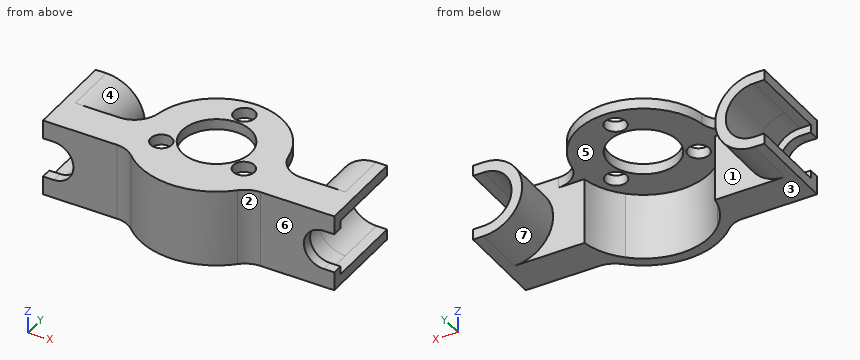
from build123d import *

# Parameters (mm, degrees)
BOSS_EXTRU_1_DEPTH      = 7
BOSS_EXTRU_3_DEPTH      = 2
ESQUISSE2_RX            = 12.5
ESQUISSE2_RY            = 12.5
ENL_V_MAT_EXTRU_1_DEPTH = 40.69604363
ESQUISSE3_R             = 12.5
ESQUISSE3_R_2           = 6.5
ESQUISSE3_R_3           = 2
BOSS_EXTRU_2_DEPTH      = 2
BOSS_EXTRU_4_DEPTH      = 14.56
CONG_2_R                = 5
BOSS_EXTRU_5_DEPTH      = 10


with BuildPart() as part:
    # Esquisse1 → Boss.-Extru.1 (new body)
    with BuildSketch(Plane(origin=(0, 0, 0), x_dir=(1, 0, 0), z_dir=(0, 1, 0))):
        with BuildLine():
            Line((36.259926639, -6.254535912), (36.259926639, -8.254535912))
            Line((36.259926639, -8.254535912), (28.259926639, -8.254535912))
            Line((28.259926639, -8.254535912), (26.259926639, -8.254535912))
            Line((26.259926639, -8.254535912), (-8.740073361, -8.254535912))
            Line((-8.740073361, -8.254535912), (-10.740073361, -8.254535912))
            Line((-10.740073361, -8.254535912), (-18.740073361, -8.254535912))
            Line((-18.740073361, -8.254535912), (-18.740073361, -6.254535912))
            Line((-18.740073361, -6.254535912), (-16.740073361, -6.254535912))
            ThreePointArc((-16.740073361, -6.254535912), (-13.378645093, -5.04629229), (-11.555635108, -1.974535912))
            ThreePointArc((-11.555635108, -1.974535912), (-11.460073361, -0.974535912), (-11.555635108, 0.025464088))
            ThreePointArc((-11.555635108, 0.025464088), (-13.378645093, 3.097220466), (-16.740073361, 4.305464088))
            Line((-16.740073361, 4.305464088), (-18.740073361, 4.305464088))
            Line((-18.740073361, 4.305464088), (-18.740073361, 6.305464088))
            Line((-18.740073361, 6.305464088), (-10.740073361, 6.305464088))
            Line((-10.740073361, 6.305464088), (-8.740073361, 6.305464088))
            Line((-8.740073361, 6.305464088), (26.259926639, 6.305464088))
            Line((26.259926639, 6.305464088), (28.259926639, 6.305464088))
            Line((28.259926639, 6.305464088), (36.259926639, 6.305464088))
            Line((36.259926639, 6.305464088), (36.259926639, 4.305464088))
            Line((36.259926639, 4.305464088), (34.259926639, 4.305464088))
            ThreePointArc((34.259926639, 4.305464088), (30.898498371, 3.097220466), (29.075488386, 0.025464088))
            ThreePointArc((29.075488386, 0.025464088), (28.979926639, -0.974535912), (29.075488386, -1.974535912))
            ThreePointArc((29.075488386, -1.974535912), (30.898498371, -5.04629229), (34.259926639, -6.254535912))
            Line((34.259926639, -6.254535912), (36.259926639, -6.254535912))
        make_face()
    extrude(amount=BOSS_EXTRU_1_DEPTH)

    # Esquisse4 → Boss.-Extru.3 (add)
    with BuildSketch(Plane.XZ):
        with BuildLine():
            Line((34.259926639, 4.724535912), (36.259926639, 4.724535912))
            Line((36.259926639, 4.724535912), (36.259926639, 6.254535912))
            Line((36.259926639, 6.254535912), (34.259926639, 6.254535912))
            ThreePointArc((34.259926639, 6.254535912), (28.979926639, 0.974535912), (34.259926639, -4.305464088))
            Line((34.259926639, -4.305464088), (36.259926639, -4.305464088))
            Line((36.259926639, -4.305464088), (36.259926639, -2.775464088))
            Line((36.259926639, -2.775464088), (34.259926639, -2.775464088))
            ThreePointArc((34.259926639, -2.775464088), (30.509926639, 0.974535912), (34.259926639, 4.724535912))
        make_face()
        with BuildLine():
            Line((-18.740073361, -2.775464088), (-18.740073361, -4.305464088))
            Line((-18.740073361, -4.305464088), (-16.740073361, -4.305464088))
            ThreePointArc((-16.740073361, -4.305464088), (-11.460073361, 0.974535912), (-16.740073361, 6.254535912))
            Line((-16.740073361, 6.254535912), (-18.740073361, 6.254535912))
            Line((-18.740073361, 6.254535912), (-18.740073361, 4.724535912))
            Line((-18.740073361, 4.724535912), (-16.740073361, 4.724535912))
            ThreePointArc((-16.740073361, 4.724535912), (-12.990073361, 0.974535912), (-16.740073361, -2.775464088))
            Line((-16.740073361, -2.775464088), (-18.740073361, -2.775464088))
        make_face()
    extrude(amount=-BOSS_EXTRU_3_DEPTH)

    # Esquisse2 → Enl_v. mat.-Extru.1 (cut, through all)
    with BuildSketch(Plane.XY.offset(8.254535912)):
        with Locations(Location((8.759926639, 9), (0, 0, 180))):
            Ellipse(ESQUISSE2_RX, ESQUISSE2_RY)
    extrude(amount=-ENL_V_MAT_EXTRU_1_DEPTH, mode=Mode.SUBTRACT)


with BuildPart() as enl_v_mat_extru_1_piece_1:
    # of the separate pieces the step leaves, piece 1, a body of its own (enl_v_mat_extru_1_pieces)
    add(part.part.solids().sort_by_distance((-18.740073361, 7, -6.305464088))[0])

    # Esquisse3 → Boss.-Extru.2 (add)
    with BuildSketch(Plane.XY.offset(8.254535912)):
        with Locations((8.759926639, 9)):
            Circle(ESQUISSE3_R)
        with Locations((8.759926639, 9)):
            Circle(ESQUISSE3_R_2, mode=Mode.SUBTRACT)
        with Locations((8.759926639, 18)):
            Circle(ESQUISSE3_R_3, mode=Mode.SUBTRACT)
        with Locations((16.554155273, 4.5)):
            Circle(ESQUISSE3_R_3, mode=Mode.SUBTRACT)
        with Locations((0.965698005, 4.5)):
            Circle(ESQUISSE3_R_3, mode=Mode.SUBTRACT)
    extrude(amount=-BOSS_EXTRU_2_DEPTH)



with BuildPart() as enl_v_mat_extru_1_piece_2:
    # of the separate pieces the step leaves, piece 2, a body of its own (enl_v_mat_extru_1_pieces)
    add(part.part.solids().sort_by_distance((34.259926639, 2, 6.254535912))[0])


with BuildPart() as enl_v_mat_extru_1_piece_1_1:
    add(enl_v_mat_extru_1_piece_1.part)

    add(enl_v_mat_extru_1_piece_2.part)  # Boss.-Extru.4 merges Enl_v. mat.-Extru.1 piece 2
    # Esquisse6 → Boss.-Extru.4 (add)
    with BuildSketch(Plane.XY.offset(8.254535912)):
        with BuildLine():
            Line((0.085250852, 0), (-2.608890362, 0))
            ThreePointArc((-2.608890362, 0), (8.759926639, -5.5), (20.12874364, 0))
            Line((20.12874364, 0), (17.434602425, 0))
            ThreePointArc((17.434602425, 0), (8.759926639, -3.5), (0.085250852, 0))
        make_face()
    extrude(amount=-BOSS_EXTRU_4_DEPTH)

    # Cong_2
    # the kernel refuses this fillet: 5 mm, written as the material it adds along each edge
    with BuildSketch(Plane(origin=(20.12874364, 0, 8.254535912), x_dir=(1, 0, 0), z_dir=(0, 0, -1))) as cong_2_piece_1:
        with BuildLine():
            CenterArc((2.20505496, 5), CONG_2_R, 225.885381452, 44.114618548)
            ThreePointArc((-1.27542503, 1.41025641), (-0.614570897, 0.726057307), (0, 0))
            Line((0, 0), (2.20505496, 0))
        make_face()
    extrude(amount=14.56)
    with BuildSketch(Plane(origin=(-2.608890362, 0, 8.254535912), x_dir=(0.6707625728642448, -0.7416721451184065, 0), z_dir=(0, 0, -1))) as cong_2_piece_2:
        with BuildLine():
            CenterArc((2.229292388, 4.989240706), CONG_2_R, 222.125947854, 44.114618548)
            Line((-1.479068338, 1.635427842), (0, 0))
            ThreePointArc((0, 0), (0.950727636, 0.031201952), (1.901455272, 0))
        make_face()
    extrude(amount=14.56)
    with BuildSketch(Plane(origin=(21.098889318, 7, 6.254535912), x_dir=(1, 0, 0), z_dir=(0, 0, 1))) as cong_2_piece_3:
        with BuildLine():
            CenterArc((4.90197697, 5), CONG_2_R, 189.870889606, 80.129110394)
            ThreePointArc((-0.024005787, 4.142857143), (0.160827475, 2.072430037), (0, 0))
            Line((0, 0), (4.90197697, 0))
        make_face()
    extrude(amount=2)
    with BuildSketch(Plane(origin=(-3.579036041, 7, 6.254535912), x_dir=(0.005794402962949308, 0.9999832123062381, 0), z_dir=(0, 0, 1))) as cong_2_piece_4:
        with BuildLine():
            CenterArc((4.971512032, 4.930866692), CONG_2_R, 180.331996692, 80.129110394)
            Line((-0.02840403, 4.901894677), (0, 0))
            ThreePointArc((0, 0), (2.071463347, 0.172833269), (4.142926693, 0))
        make_face()
    extrude(amount=2)

    # Esquisse7 → Boss.-Extru.5 (add)
    with BuildSketch(Plane(origin=(0, 7, 0), x_dir=(1, 0, 0), z_dir=(0, 1, 0))):
        with BuildLine():
            Line((36.259926639, -8.254535912), (36.259926639, -6.254535912))
            Line((36.259926639, -6.254535912), (34.259926639, -6.254535912))
            ThreePointArc((34.259926639, -6.254535912), (28.979926639, -0.974535912), (34.259926639, 4.305464088))
            Line((34.259926639, 4.305464088), (36.259926639, 4.305464088))
            Line((36.259926639, 4.305464088), (36.259926639, 6.305464088))
            Line((36.259926639, 6.305464088), (34.259926639, 6.305464088))
            ThreePointArc((34.259926639, 6.305464088), (26.979926639, -0.974535912), (34.259926639, -8.254535912))
            Line((34.259926639, -8.254535912), (36.259926639, -8.254535912))
        make_face()
        with BuildLine():
            Line((-18.740073361, 6.305464088), (-16.740073361, 6.305464088))
            ThreePointArc((-16.740073361, 6.305464088), (-9.460073361, -0.974535912), (-16.740073361, -8.254535912))
            Line((-16.740073361, -8.254535912), (-18.740073361, -8.254535912))
            Line((-18.740073361, -8.254535912), (-18.740073361, -6.254535912))
            Line((-18.740073361, -6.254535912), (-16.740073361, -6.254535912))
            ThreePointArc((-16.740073361, -6.254535912), (-11.460073361, -0.974535912), (-16.740073361, 4.305464088))
            Line((-16.740073361, 4.305464088), (-18.740073361, 4.305464088))
            Line((-18.740073361, 4.305464088), (-18.740073361, 6.305464088))
        make_face()
    extrude(amount=BOSS_EXTRU_5_DEPTH)


solid = enl_v_mat_extru_1_piece_1_1.part
Read the model definition and answer for the solid it produces. Units are mm, in the model's axes. Face numbers are marked on the shaded views. A direction names the side the tool comes from. Give positions to 0.01 mm unless a question says otherwise; leave off trailing zeros. Loops run counter-clockwise (first coordinate to the right, second up) from the corner with the lowest first, then second, coordinate; pieces in that order, holes last. Notation, with made-up numbers: (54.25, -9) -> (93.25, -9) arc R24 ccw to (93.25, 21) -> close; hole circle Ø10 at (78.5, 51). An arc over 180 degrees is marked (long way). Answer as CSV lines item,"result".
Item 1: Find section D-D on x = 28. Give the vertices of the cut face in (y, z).
Returned:
outline,"(0, -6.31) -> (7, -6.31) -> (7, -2.74) -> (17, -2.74) -> (17, 4.69) -> (7, 4.69) -> (7, 8.25) -> (0, 8.25) -> close"
Item 2: Consider line 1 (Y direction, x = -9, z = -4); line 2 (Z direction, x = -12.5, y = 8.5); line 3 (X direction, y = 12.5, z = 1.5). Determine where each line is inside the solid, lowest interval first. Write a range as [from, to].
Returned:
line 1,"y = [0, 7]"
line 2,"z = [-4.94, -2.17], [4.12, 6.89]"
line 3,"x = [-11.49, -9.48], [27, 29.01]"
Item 3: Find section B-B on x = -14.5. Give the vertices of the cut face in (y, z), plus the area to 3 significant figures.
Returned:
outline,"(0, -6.31) -> (7, -6.31) -> (7, -5.95) -> (17, -5.95) -> (17, -3.81) -> (2, -3.81) -> (2, -2.03) -> (0, -2.03) -> close; (0, 3.98) -> (2, 3.98) -> (2, 5.76) -> (17, 5.76) -> (17, 7.9) -> (7, 7.9) -> (7, 8.25) -> (0, 8.25) -> close"
area,"85.0 mm²"
Item 4: Find section C-C on y = 9. Give the vertices of the cut face in (x, z).
Returned:
outline,"(-18.74, -6.31) -> (-16.74, -6.31) arc R7.28 ccw to (-16.74, 8.25) -> (-18.74, 8.25) -> (-18.74, 6.25) -> (-16.74, 6.25) arc R5.28 cw to (-16.74, -4.31) -> (-18.74, -4.31) -> close; (-4.48, 6.25) -> (2.26, 6.25) -> (2.26, 8.25) -> (-4.48, 8.25) -> close; (15.26, 6.25) -> (22, 6.25) -> (22, 8.25) -> (15.26, 8.25) -> close; (34.26, -6.31) -> (36.26, -6.31) -> (36.26, -4.31) -> (34.26, -4.31) arc R5.28 cw to (34.26, 6.25) -> (36.26, 6.25) -> (36.26, 8.25) -> (34.26, 8.25) arc R7.28 ccw to start"
Item 5: Determine the mould class of the marked faces 1, 2, 3 and 4 for opening direction X: +X half, -X half, draft (parallel to the pull), parting line (faces both ways), or undercut.
Returned:
face 1,"undercut"
face 2,"+X half"
face 3,"draft"
face 4,"undercut"
Item 6: Find section A-A on y = 18. Give the vertices of the cut face in (x, z), plus the area to 3 significant figures.
Returned:
outline,"(0.09, 6.25) -> (6.76, 6.25) -> (6.76, 8.25) -> (0.09, 8.25) -> close; (10.76, 6.25) -> (17.43, 6.25) -> (17.43, 8.25) -> (10.76, 8.25) -> close"
area,"26.7 mm²"
Item 7: For the marked faces 5, 6 and 7, determine the directions among +Z, -Z, +X, -X, +Y, -Y from which every point of the face is accessible in a straight line to the end or side of a thin tool.
Returned:
face 5,"-Z, +Y"
face 6,"+Z, -Z, +X, -Y"
face 7,"+Y"
Item 8: Each of these flat-tipped pins is pushed along its axis until it touches: pin 1 (6 mm diameter, centred on x = 15.5, z = -2.5, fed in from +Y); pin 2 (8 mm diameter, centred on x = 8.76, y = 9, fed in from +Z); pin 3 (12.5 mm diameter, centred on x = 2.5, y = 14.5, fed in from -Z); pin 4 (1 mm diameter, centred on y = 10, z = 4, fed in from -X). Where does it stop, or does it pass through?
Returned:
pin 1,"stops at y = 1.17"
pin 2,"passes through"
pin 3,"stops at z = 6.25"
pin 4,"stops at x = -12.81"
